Check sheet for the drawn part. Datum: minimum x, y, z corner. Units: mm. Round coordinates to 2 decimals unless told otherwise and drop trailing zeros. Order: outer loops, then holes, each group sorted by start corner. A loop starts at its lowest first (then second) coordinate and runs counter-clockwise, first axis right, second up.
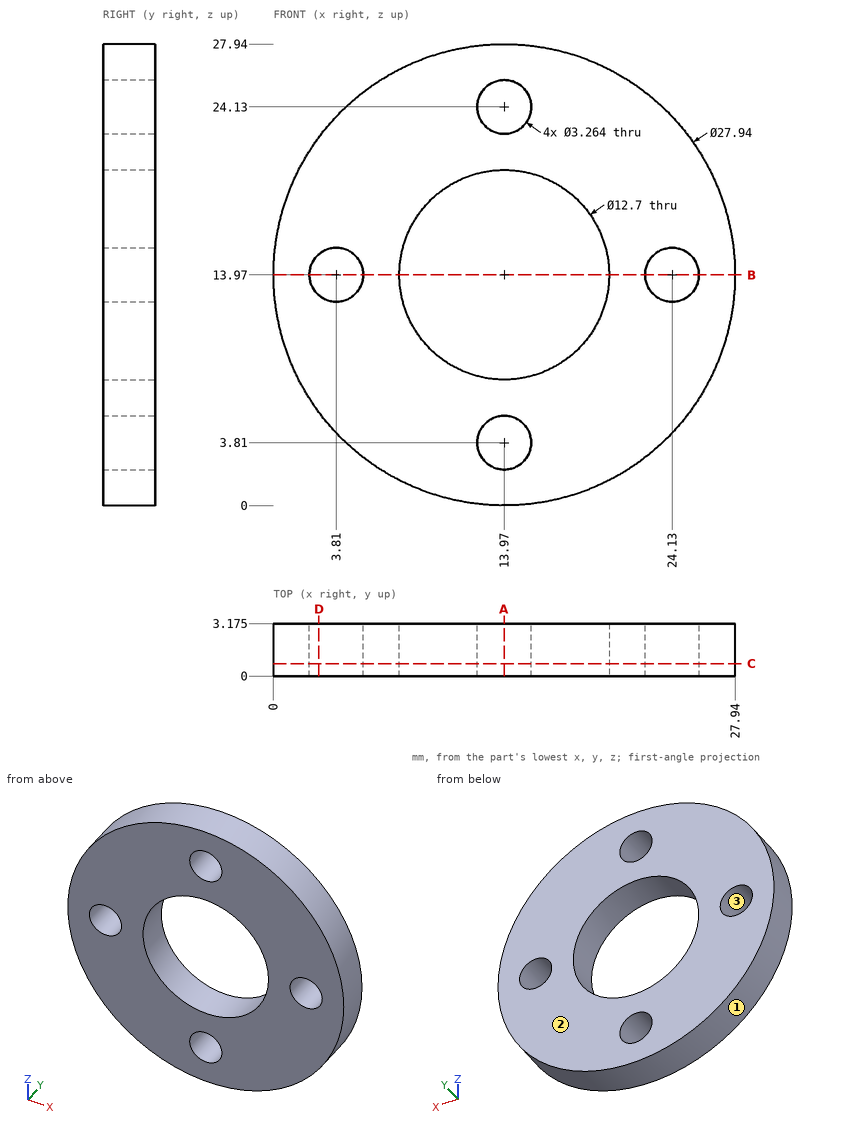
1) Scan lines: line 1 (Z direction, x = 13.97, y = 2.15); line 2 (Z direction, x = 3, y = 3). Record each from-to range of solid material in increasing order.
2) Sectioned sample at D-D on x = 2.75. Record the cut outline in (y, z) (3 decimals).
3) Gauge pin test, flat end, axial feed: pin 1 (1.5 mm diameter, centred on x = 18, y = 1, fed in from -Z). Record the tip position at first contact, or that the pin passes through.
4) Sectioned sample at A-A on x = 13.97. Record the cut outline in (y, z) (3 decimals).
5) Sectioned sample at B-B on z = 13.97. Record the cut outline in (x, y) (3 decimals).
6) Sectioned sample at C-C on y = 0.75. Record the cut outline in (x, z), and give its area (3 significant figures).
7) Draft check along Z on the marked faces 1, 2 and 3. Enter one of: pulls with the +Z half, pulls with the -Z half, needs draft (parallel to the pull), parting line crosses it, or undercut.
Values found:
1. line 1: z = 0 to 2.18, 5.44 to 7.62, 20.32 to 22.5, 25.76 to 27.94
1. line 2: z = 5.32 to 12.55, 15.39 to 22.62
2. outline: (0, 5.647) - (3.175, 5.647) - (3.175, 12.729) - (0, 12.729) - close; (0, 15.211) - (3.175, 15.211) - (3.175, 22.293) - (0, 22.293) - close
3. pin 1: stops at z = 0.39
4. outline: (0, 0) - (3.175, 0) - (3.175, 2.178) - (0, 2.178) - close; (0, 5.442) - (3.175, 5.442) - (3.175, 7.62) - (0, 7.62) - close; (0, 20.32) - (3.175, 20.32) - (3.175, 22.498) - (0, 22.498) - close; (0, 25.762) - (3.175, 25.762) - (3.175, 27.94) - (0, 27.94) - close
5. outline: (0, 0) - (2.178, 0) - (2.178, 3.175) - (0, 3.175) - close; (5.442, 0) - (7.62, 0) - (7.62, 3.175) - (5.442, 3.175) - close; (20.32, 0) - (22.498, 0) - (22.498, 3.175) - (20.32, 3.175) - close; (25.762, 0) - (27.94, 0) - (27.94, 3.175) - (25.762, 3.175) - close
6. outline: circle Ø27.94 at (13.97, 13.97); hole circle Ø3.26 at (3.81, 13.97); hole circle Ø12.7 at (13.97, 13.97); hole circle Ø3.26 at (13.97, 3.81); hole circle Ø3.26 at (13.97, 24.13); hole circle Ø3.26 at (24.13, 13.97)
6. area: 453 mm2
7. face 1: parting line crosses it
7. face 2: needs draft
7. face 3: undercut
